Design review of the part built by this model. Coordinates are the model's own, in mm. Face numbers are marked on the shaded views. A direction names the side the tool comes from. Round coordinates to 2 decimals unless told otherwise and drop trailing zeros. Write each loop counter-clockwise with the first axis right and the second up, starting at its lowest first coordinate (ties: lowest second). Pieces come first, ordered by that corner, then holes.
from build123d import *


with BuildPart() as part:
    # Croquis1 → Revoluci_n1 (revolve)
    with BuildSketch(Plane.XY, mode=Mode.PRIVATE) as revoluci_n1_sk:
        with BuildLine():
            Line((-2, 4.019010036), (-2, 1))
            ThreePointArc((-2, 1), (-1.707106781, 0.292893219), (-1, 0))
            Line((-1, 0), (0, 0))
            Line((0, 0), (0, 8))
            ThreePointArc((0, 8), (-2.395650681, 7.632880047), (-4.571428571, 6.565214453))
            ThreePointArc((-4.571428571, 6.565214453), (-4.97267486, 5.512391122), (-4.139173101, 4.754294578))
            Line((-4.139173101, 4.754294578), (-2.43041345, 4.51414407))
            ThreePointArc((-2.43041345, 4.51414407), (-2.12264521, 4.34703955), (-2, 4.019010036))
        make_face()
    revolve(revoluci_n1_sk.sketch.rotate(Axis((0, 0, 0), (0, 1, 0)), 270), axis=Axis((0, 0, 0), (0, 1, 0)))


solid = part.part
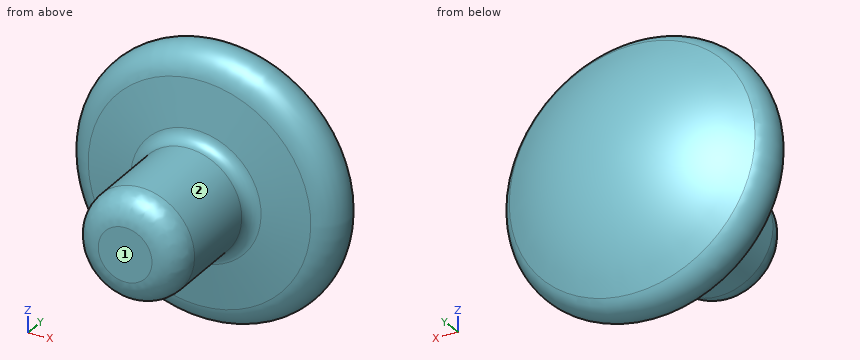
1) For P1, Ø1.5, axis at x = -2.5, y = 2, coming from the +Z side; P2, Ø4, axis at x = 0.5, y = 2, coming from the +Z side, all flat-tipped, find the tip position at first contact; note any pin that passes through.
2) For line 1 along Z through (x, y) = (1.25, 2); line 2 along Z through (x, y) = (3, 5); line 3 along Y through (x, z) = (3, -1.75), list the stretches that pass through material, from the lowest coordinate up.
3) Add section B-B on y = 7. State the section outline as (x, z) points, and give its area (3 significant figures).
4) Add section A-A on y = 2.75. State the section outline as (x, z) points.
5) For the marked faces 1 and 2, list the 3-axis set-ups (+Z, -Z, +X, -X, +Y, -Y) from which the entire face can be reached by the end or side of a thin tool; tool diameter is ignored.
Computed:
1. P1: stops at z = 0.97
1. P2: stops at z = 2
2. line 1: z = -1.56 to 1.56
2. line 2: z = -3.58 to 3.58
2. line 3: y = 4.66 to 7.21
3. outline: circle Ø7.75 at (0, 0)
3. area: 47.1 mm2
4. outline: circle Ø4 at (0, 0)
5. face 1: +Z, -Z, +X, -X, -Y
5. face 2: -Y
